Geometry: final body of the model. Coordinates: model frame, mm. A direction names the side the tool comes from. Coordinates: 2 decimals unless noted, no trailing zeros. Loops run counter-clockwise (first coordinate to the right, second up) from the corner with the lowest first, then second, coordinate; pieces in that order, holes last. Notation, with made-up numbers: (43, 78) - (57, 78) arc R21 cw to (57, 103) - close; hole circle Ø1 at (13, 85). An arc over 180 degrees is marked (long way). Put each result on its own line as item: value. Start each with the question number.
1) Section D-D on x = -20. Output: boundary loops of the cut face in (y, z), and give its area (3 significant figures).
2) Section B-B on y = 0. Count the separate pieces of the cut face and the enclosed holes in it, and give its area (3 significant figures).
3) Section A-A on z = 0. Output: boundary loops of the cut face in (x, y).
4) Contact query for flat-ended pins moving along their axis: pin 1 Ø5.5 at (y, z) = (47.24, -47.24) entering from -X; pin 2 Ø16.5 at (y, z) = (0, -41.275) entering from -X; pin 3 Ø20 at (y, z) = (7.5, 9) entering from +X; pin 4 Ø3 at (y, z) = (-4, -15) entering from +X. Output: stop coordinate, or through.
5) Material intervals for line 1 along Y through (x, z) = (-6, -45); line 2 along X through (y, z) = (66, -21); line 3 along Y through (x, z) = (-10, 4), sorted ascending. Write a range as from..to.
6) Reachability of faces 1 (the flat face through (-10.16, 16, -16)), 2 (the cylindrical face through (-1.88, 13.6, 17.74)), 3 (the cylindrical face through (-5.01, -44.72, -49.17)) from +Z, -Z, +X, -X, +Y, -Y: full face, straight path, thin tool, end or side. Return the list, or none.
7) Draft query along Z for faces 4 (the cylindrical face through (-5.151, 74.388, 16.519)), 5 (the flat face through (0, 16, 16)), 6 (the cylindrical face through (-5.01, -63.63, -0.14)). Return one class per face: +Z half, -Z half, draft (parallel to the pull), parting line (faces both ways), or undercut.
8) Section C-C on z = 42. Output: boundary loops of the cut face in (x, y), and give its area (3 significant figures).
```python
from build123d import *

# Parameters (mm, degrees)
CUT_EXTRUDE1_DEPTH      = 113.342968182
CUT_EXTRUDE1_DEPTH_BACK = 113.342968182
SKETCH2_R               = 6.35
SKETCH3_R               = 3.175
CUT_EXTRUDE2_DEPTH      = 113.342968182
CIRPATTERN1_COUNT       = 8


with BuildPart() as part:
    # Sketch1 → Revolve1 (revolve)
    with BuildSketch(Plane.XY, mode=Mode.PRIVATE) as revolve1_sk:
        with BuildLine():
            Line((0, 76.2), (-10.16, 76.2))
            Line((-10.16, 76.2), (-10.16, 21.082))
            ThreePointArc((-10.16, 21.082), (-11.647897552, 17.489897552), (-15.24, 16.002))
            Line((-15.24, 16.002), (-31.75, 16.002))
            Line((-31.75, 16.002), (-31.75, 9.652))
            Line((-31.75, 9.652), (-6.35, 9.652))
            Line((-6.35, 9.652), (-6.35, 19.812))
            ThreePointArc((-6.35, 19.812), (-5.606051224, 21.608051224), (-3.81, 22.352))
            Line((-3.81, 22.352), (0, 22.352))
            Line((0, 22.352), (0, 76.2))
        make_face()
    revolve(revolve1_sk.sketch.rotate(Axis((0, 0, 0), (-1, 0, 0)), 90), axis=Axis((0, 0, 0), (-1, 0, 0)))

    # Sketch2 → Cut-Extrude1 (cut, two sides: drawn at the far end of the back side and taken through both)
    with BuildSketch(Plane(origin=(0, 0, 0), x_dir=(0, 0, -1), z_dir=(1, 0, 0)).offset(-CUT_EXTRUDE1_DEPTH_BACK)):
        with Locations((41.275, 0)):
            Circle(SKETCH2_R)
        with Locations((-41.275, 0)):
            Circle(SKETCH2_R)
    extrude(amount=CUT_EXTRUDE1_DEPTH + CUT_EXTRUDE1_DEPTH_BACK, mode=Mode.SUBTRACT)

    # Sketch3 → Cut-Extrude2 (cut, through all)
    with BuildSketch(Plane(origin=(0, 0, 0), x_dir=(0, 0, -1), z_dir=(1, 0, 0))):
        with Locations((66.802, 0)):
            Circle(SKETCH3_R)
    cut_extrude2 = extrude(amount=-CUT_EXTRUDE2_DEPTH, mode=Mode.SUBTRACT)

    # CirPattern1: Cut-Extrude2 ×8 about axis
    cirpattern1_axis = Axis((0, 0, 0), (1, 0, 0))
    for i in range(1, CIRPATTERN1_COUNT):
        add(cut_extrude2.rotate(cirpattern1_axis, i * 360 / CIRPATTERN1_COUNT), mode=Mode.SUBTRACT)


solid = part.part
```
Answer block:
1. outline: circle Ø32 at (0, 0); hole circle Ø19.3 at (0, 0)
1. area: 512 mm²
2. separate pieces: 6
2. enclosed holes: 0
2. area: 1,090 mm²
3. outline: (-31.75, -16) - (-15.24, -16) arc R5.08 cw to (-10.16, -21.08) - (-10.16, -63.63) - (0, -63.63) - (0, -22.35) - (-3.81, -22.35) arc R2.54 cw to (-6.35, -19.81) - (-6.35, -9.65) - (-31.75, -9.65) - close; (-31.75, 9.65) - (-6.35, 9.65) - (-6.35, 19.81) arc R2.54 cw to (-3.81, 22.35) - (0, 22.35) - (0, 63.63) - (-10.16, 63.63) - (-10.16, 21.08) arc R5.08 cw to (-15.24, 16) - (-31.75, 16) - close; (-10.16, -76.2) - (0, -76.2) - (0, -69.98) - (-10.16, -69.98) - close; (-10.16, 69.98) - (0, 69.98) - (0, 76.2) - (-10.16, 76.2) - close
4. pin 1: passes through
4. pin 2: stops at x = -10.16
4. pin 3: stops at x = -5.49
4. pin 4: stops at x = -6.35
5. line 1: y = -61.49..-49.49, -44.98..-5.14, 5.14..44.98, 49.49..61.49
5. line 2: x = -10.16..0
5. line 3: y = -76.09..-8.78, 8.78..76.09
6. face 1: -X
6. face 2: +X
6. face 3: +X, -X
7. face 4: parting line
7. face 5: draft
7. face 6: undercut
8. outline: (-10.16, -63.58) - (0, -63.58) - (0, -6.31) - (-10.16, -6.31) - close; (-10.16, 6.31) - (0, 6.31) - (0, 63.58) - (-10.16, 63.58) - close
8. area: 1,160 mm²
